from build123d import *

# Parameters (mm, degrees)
SKETCH_R      = 8
PAD_DEPTH     = 5
SKETCH001_R   = 10
SKETCH001_R_2 = 6
PAD001_DEPTH  = 2
PAD002_DEPTH  = 2


with BuildPart() as part:
    # Sketch → Pad (new body)
    with BuildSketch(Plane.XY):
        with BuildLine():
            ThreePointArc((-2.142857, -9.76771), (10, 0), (-2.142857, 9.76771))
            Line((-28.857143, 3.907084), (-2.142857, 9.76771))
            ThreePointArc((-28.857143, 3.907084), (-32, 0), (-28.857143, -3.907084))
            Line((-2.142857, -9.76771), (-28.857143, -3.907084))
        make_face()
        Circle(SKETCH_R, mode=Mode.SUBTRACT)
    extrude(amount=PAD_DEPTH)

    # Sketch001 (on Face7 of Pad) → Pad001 (join)
    with BuildSketch(Plane.XY.offset(5)):
        Circle(SKETCH001_R)
        Circle(SKETCH001_R_2, mode=Mode.SUBTRACT)
    extrude(amount=PAD001_DEPTH)

    # Sketch002 (on Face7 of Pad001) → Pad002 (join)
    with BuildSketch(Plane.XY.offset(5)):
        with BuildLine():
            ThreePointArc((-28.857143, 3.907084), (-32, 0), (-28.857143, -3.907084))
            Line((-28.857143, -3.907084), (-22.089875, -5.391699))
            ThreePointArc((-22.089875, -5.391699), (-20, 0), (-22.089875, 5.391699))
            Line((-28.857143, 3.907084), (-22.089875, 5.391699))
        make_face()
    extrude(amount=PAD002_DEPTH)


solid = part.part
The listing builds one solid part. Answer for the finished solid, in the listing's coordinates (mm). A direction names the side the tool comes from. Give positions to 0.01 mm unless a question says otherwise; leave off trailing zeros. Write each loop counter-clockwise with the first axis right and the second up, starting at its lowest first coordinate (ties: lowest second). Pieces come first, ordered by that corner, then holes.
Item 1: Section B-B, the plane x = 0 is taken. Write down the section's boundary in (y, z).
Item 2: Determine the mould class of faces 1 (the flat face through (0, -7, 7)), 2 (the cylindrical face through (-6, 0, 6)), 3 (the cylindrical face through (-32, 0, 3)) for opening direction Y: released by +Y, released by -Y, zero draft, split by the parting line, or undercut.
Item 3: Section A-A, the plane y = 0 is taken. Write down the section's boundary in (x, z), plus the area to 3 significant figures.
Item 4: Section C-C, the plane z = 3.5 is taken. Write down the section's boundary in (x, y), plus the area to 3 significant figures.
Item 5: Section D-D, the plane y = -7 is taken. Write down the section's boundary in (x, z).
Item 6: Which of the six approach directions +Z, -Z, +X, -X, +Y, -Y give full straight-line access (tool end or side, diameter ignored) to faces 4 (the cylindrical face through (-1.73, -7.81, 2.46)), 5 (the cylindrical face through (-20, 0, 6)), 6 (the flat face through (-26, 0, 7))?
Item 7: Flat-ended cylindrical pins translate along their axes: P1, Ø5, axis at x = 0, y = 3, coming from the -Z side; P2, Ø3, axis at x = -15, y = -7, coming from the +Z side; P3, Ø3, axis at y = 3, z = 3, coming from the +X side. Find the tip coordinate at first contact, or state that the pin passes through.
Item 8: Find the intervals of material crossed by line 1 along Y through (x, z) = (0, 5.6); line 2 along Y through (x, z) = (0, 2.75); line 3 along X through (y, z) = (-2.5, 5.25), in increasing order.
Completed:
1. outline: (-10, 0) - (-8, 0) - (-8, 5) - (-6, 5) - (-6, 7) - (-10, 7) - close; (6, 5) - (8, 5) - (8, 0) - (10, 0) - (10, 7) - (6, 7) - close
2. face 1: zero draft
2. face 2: undercut
2. face 3: split by the parting line
3. outline: (-32, 0) - (-8, 0) - (-8, 5) - (-6, 5) - (-6, 7) - (-10, 7) - (-10, 5) - (-20, 5) - (-20, 7) - (-32, 7) - close; (6, 5) - (8, 5) - (8, 0) - (10, 0) - (10, 7) - (6, 7) - close
3. area: 170 mm2
4. outline: (-28.86, -3.91) - (-2.14, -9.77) arc R10 ccw (long way) to (-2.14, 9.77) - (-28.86, 3.91) arc R4 ccw to start; hole circle Ø16 at (0, 0)
4. area: 382 mm2
5. outline: (-14.76, 0) - (-3.87, 0) - (-3.87, 5) - (3.87, 5) - (3.87, 0) - (7.14, 0) - (7.14, 7) - (-7.14, 7) - (-7.14, 5) - (-14.76, 5) - close
6. face 4: -Z
6. face 5: +Z
6. face 6: +Z, +X, -X, +Y, -Y
7. P1: passes through
7. P2: stops at z = 5
7. P3: stops at x = 9.89
8. line 1: y = -10 to -6, 6 to 10
8. line 2: y = -10 to -8, 8 to 10
8. line 3: x = -31.12 to -20.4, -9.68 to -5.45, 5.45 to 9.68
